from build123d import *

# Parameters (mm, degrees)
SKETCH1_W               = 93
SKETCH1_H               = 58
BOSS_EXTRUDE1_DEPTH     = 3
SKETCH2_R               = 1.5
CUT_EXTRUDE2_DEPTH      = 3
CUT_EXTRUDE3_DEPTH      = 10
CUT_EXTRUDE3_DEPTH_BACK = 10
SKETCH6_W               = 23
SKETCH6_H               = 45
CUT_EXTRUDE4_DEPTH      = 10
SKETCH7_W               = 93
SKETCH7_H               = 6.5
BOSS_EXTRUDE2_DEPTH     = 3
SKETCH8_R               = 6.5
SKETCH8_W               = 6.5
SKETCH8_H               = 6.5
BOSS_EXTRUDE3_DEPTH     = 3
SKETCH9_R               = 2
CUT_EXTRUDE6_DEPTH      = 4
SKETCH12_R              = 6.5
SKETCH12_R_2            = 2
BOSS_EXTRUDE5_DEPTH     = 3
SKETCH14_R              = 2
CUT_EXTRUDE7_DEPTH      = 10


with BuildPart() as part:
    # Sketch1 → Boss-Extrude1 (new body)
    with BuildSketch(Plane.XY):
        Rectangle(SKETCH1_W, SKETCH1_H)
    extrude(amount=BOSS_EXTRUDE1_DEPTH)

    # Sketch2 → Cut-Extrude2 (cut)
    with BuildSketch(Plane.XY.offset(3)):
        with BuildLine():
            ThreePointArc((-42.5, 26.5), (-43.560660172, 26.060660172), (-44, 25))
            Line((-44, 25), (-42.5, 25))
            Line((-42.5, 25), (-42.5, 26.5))
        make_face()
        with BuildLine():
            Line((-42.5, 25), (-44, 25))
            ThreePointArc((-44, 25), (-42.5, 23.5), (-41, 25))
            ThreePointArc((-41, 25), (-41.439339828, 26.060660172), (-42.5, 26.5))
            Line((-42.5, 26.5), (-42.5, 25))
        make_face()
        with Locations((-42.5, -25)):
            Circle(SKETCH2_R)
        with Locations((42.5, -25)):
            Circle(SKETCH2_R)
        with Locations((42.5, 25)):
            Circle(SKETCH2_R)
    extrude(amount=-CUT_EXTRUDE2_DEPTH, mode=Mode.SUBTRACT)

    # Sketch5 → Cut-Extrude3 (cut, two sides)
    with BuildSketch(Plane.XY.offset(3)) as cut_extrude3_sk:
        with BuildLine():
            ThreePointArc((-36.5, 22.5), (-37.903805922, 20.403805922), (-40, 19))
            Line((-40, 19), (-40, -19))
            ThreePointArc((-40, -19), (-37.903805922, -20.403805922), (-36.5, -22.5))
            Line((-36.5, -22.5), (-15.5, -22.5))
            Line((-15.5, -22.5), (-15.5, 22.5))
            Line((-15.5, 22.5), (-36.5, 22.5))
        make_face()
        with BuildLine():
            Line((20.5, -22.5), (36.5, -22.5))
            ThreePointArc((36.5, -22.5), (37.903805922, -20.403805922), (40, -19))
            Line((40, -19), (40, 19))
            ThreePointArc((40, 19), (37.903805922, 20.403805922), (36.5, 22.5))
            Line((36.5, 22.5), (20.5, 22.5))
            Line((20.5, 22.5), (20.5, -22.5))
        make_face()
    extrude(amount=CUT_EXTRUDE3_DEPTH, mode=Mode.SUBTRACT)
    extrude(cut_extrude3_sk.sketch, amount=-CUT_EXTRUDE3_DEPTH_BACK, mode=Mode.SUBTRACT)

    # Sketch6 → Cut-Extrude4 (cut)
    with BuildSketch(Plane.XY.offset(3)):
        with Locations((2.5, 0)):
            Rectangle(SKETCH6_W, SKETCH6_H)
    extrude(amount=-CUT_EXTRUDE4_DEPTH, mode=Mode.SUBTRACT)

    # Sketch7 → Boss-Extrude2 (add, through all)
    with BuildSketch(Plane.XY.offset(3)):
        Rectangle(SKETCH7_W, SKETCH7_H)
    extrude(amount=-BOSS_EXTRUDE2_DEPTH)

    # Sketch8 → Boss-Extrude3 (add, through all)
    with BuildSketch(Plane.XY.offset(3)):
        with Locations((-12.25, 0)):
            Circle(SKETCH8_R)
        with Locations((-12.25, 0)):
            Rectangle(SKETCH8_W, SKETCH8_H, mode=Mode.SUBTRACT)
        with Locations((17.25, 0)):
            Circle(SKETCH8_R)
        with Locations((17.25, 0)):
            Rectangle(SKETCH8_W, SKETCH8_H, mode=Mode.SUBTRACT)
    extrude(amount=-BOSS_EXTRUDE3_DEPTH)

    # Sketch9 → Cut-Extrude6 (cut, through all)
    with BuildSketch(Plane.XY.offset(3)):
        with Locations((-12.000998453, 0)):
            Circle(SKETCH9_R)
        with Locations((17.999001547, 0)):
            Circle(SKETCH9_R)
    extrude(amount=-CUT_EXTRUDE6_DEPTH, mode=Mode.SUBTRACT)

    # Sketch12 → Boss-Extrude5 (add, through all)
    with BuildSketch(Plane.XY.offset(3)):
        with Locations((-32, 0)):
            Circle(SKETCH12_R)
        with Locations((-32, 0)):
            Circle(SKETCH12_R_2, mode=Mode.SUBTRACT)
    extrude(amount=-BOSS_EXTRUDE5_DEPTH)

    # Sketch14 → Cut-Extrude7 (cut)
    with BuildSketch(Plane.XY.offset(3)):
        with Locations((-32.000998453, 0)):
            Circle(SKETCH14_R)
    extrude(amount=-CUT_EXTRUDE7_DEPTH, mode=Mode.SUBTRACT)


solid = part.part
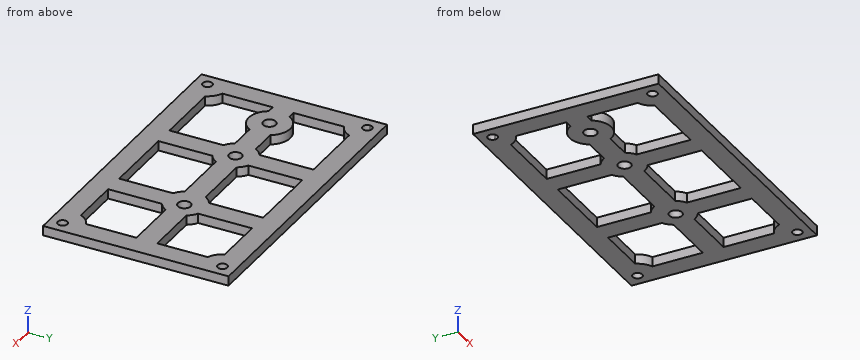
For this review, take the finished solid that the model builds, in its own axes (mm). Give positions to 0.01 mm unless a question says otherwise; leave off trailing zeros. Loops run counter-clockwise (first coordinate to the right, second up) from the corner with the lowest first, then second, coordinate; pieces in that order, holes last. Notation, with made-up numbers: M -30.5,55.5 L -1.5,55.5 A15 ccw -1.5,70.5 Z; hole C 79,-37.75 d1. An arc over 180 degrees is marked long. Answer as a JSON object with one key per item and string values. Group by question number.
Q1. Add section A-A on y = -25. Give the boundary of the cut face in (x, z), and give its area (3 significant figures).
Q2. For probe 1 along Y at (x, z) = (6, 2.15); probe 2 along X at (y, z) = (7, 1.6); probe 3 along Y at (x, z) = (42.5, 1.45), list the stretches that pass through material, from the lowest coordinate up. Write a range as [from, to].
Q3. Add section B-B on x = 26. Give the boundary of the cut face in (y, z), and give its area (3 significant figures).
Q4. Add section C-C on y = 0. Give the boundary of the cut face in (x, z), and give its area (3 significant figures).
Q5. Add section D-D on x = -13. Give the boundary of the cut face in (y, z), and give its area (3 significant figures).
Q6. Insertion check: P1, Ø3.5, axis at x = 42.5, y = 25, coming from the +Z side. The pin has a flat end and moves straight along its axis. Give the tip position at first contact, or say it passes through.
Checked values:
{
 "1": {"outline": "M -46.5,0 L -44,0 L -44,3 L -46.5,3 Z; M -41,0 L 41,0 L 41,3 L -41,3 Z; M 44,0 L 46.5,0 L 46.5,3 L 44,3 Z", "area": "261 mm²"},
 "2": {"probe 1": "[-29, -22.5], [-3.25, 3.25], [22.5, 29]", "probe 2": "[-46.5, -40], [-15.5, -9], [14, 20.5], [40, 46.5]", "probe 3": "[-29, -26.5], [-23.5, 23.5], [26.5, 29]"},
 "3": {"outline": "M -29,0 L -22.5,0 L -22.5,3 L -29,3 Z; M -3.25,0 L 3.25,0 L 3.25,3 L -3.25,3 Z; M 22.5,0 L 29,0 L 29,3 L 22.5,3 Z", "area": "58.5 mm²"},
 "4": {"outline": "M -46.5,0 L -34,0 L -34,3 L -46.5,3 Z; M -30,0 L -14,0 L -14,3 L -30,3 Z; M -10,0 L 16,0 L 16,3 L -10,3 Z; M 20,0 L 46.5,0 L 46.5,3 L 20,3 Z", "area": "243 mm²"},
 "5": {"outline": "M -29,0 L -1.73,0 L -1.73,3 L -29,3 Z; M 1.73,0 L 29,0 L 29,3 L 1.73,3 Z", "area": "164 mm²"},
 "6": {"P1": "z = 3"}
}
